Design review of the part built by this model. Coordinates are the model's own, in mm. A direction names the side the tool comes from. Round coordinates to 2 decimals unless told otherwise and drop trailing zeros. Order: outer loops, then holes, each group sorted by start corner. A loop starts at its lowest first (then second) coordinate and runs counter-clockwise, first axis right, second up. Notation, with made-up numbers: (10.5, 4.25) - (15.5, 4.25) arc R25 ccw to (15.5, 38.25) - close; hole circle Ø8 at (-11, 46.5). An arc over 180 degrees is marked (long way). Use CSV: the item, a comma, the result in double quotes.
from build123d import *

# Parameters (mm, degrees)
SKETCH_2_R          = 1.3
EXTRUDE_2_DEPTH     = 3
SKETCH_4_W          = 2
SKETCH_4_H          = 4
EXTRUDE_3_DEPTH     = 6
SKETCH_6_R          = 1.1
CUT_EXTRUDE_2_DEPTH = 45.75


with BuildPart() as part:
    # 草图2 → 凸台-拉伸2 (new body)
    with BuildSketch(Plane.XY):
        with BuildLine():
            ThreePointArc((-3.5, -10), (-2.767766953, -11.767766953), (-1, -12.5))
            Line((-1, -12.5), (50, -12.5))
            ThreePointArc((50, -12.5), (51.767766953, -11.767766953), (52.5, -10))
            Line((52.5, -10), (52.5, 1))
            ThreePointArc((52.5, 1), (51.767766953, 2.767766953), (50, 3.5))
            Line((50, 3.5), (-1, 3.5))
            ThreePointArc((-1, 3.5), (-2.767766953, 2.767766953), (-3.5, 1))
            Line((-3.5, 1), (-3.5, -10))
        make_face()
        with Locations((0, -9)):
            Circle(SKETCH_2_R, mode=Mode.SUBTRACT)
        Circle(SKETCH_2_R, mode=Mode.SUBTRACT)
        with Locations((49, -9)):
            Circle(SKETCH_2_R, mode=Mode.SUBTRACT)
        with Locations((49, 0)):
            Circle(SKETCH_2_R, mode=Mode.SUBTRACT)
    extrude(amount=EXTRUDE_2_DEPTH)

    # 草图4 → 凸台-拉伸3 (add)
    with BuildSketch(Plane.XY.offset(3)):
        with Locations((8.75, 1.5)):
            Rectangle(SKETCH_4_W, SKETCH_4_H)
        with Locations((13.25, 1.5)):
            Rectangle(SKETCH_4_W, SKETCH_4_H)
        with Locations((35.75, 1.5)):
            Rectangle(SKETCH_4_W, SKETCH_4_H)
        with Locations((40.25, 1.5)):
            Rectangle(SKETCH_4_W, SKETCH_4_H)
        with Locations((11.25, -10.5)):
            Rectangle(SKETCH_4_W, SKETCH_4_H)
        with Locations((15.75, -10.5)):
            Rectangle(SKETCH_4_W, SKETCH_4_H)
        with Locations((33.25, -10.5)):
            Rectangle(SKETCH_4_W, SKETCH_4_H)
        with Locations((37.75, -10.5)):
            Rectangle(SKETCH_4_W, SKETCH_4_H)
    extrude(amount=EXTRUDE_3_DEPTH)

    # 草图6 → 切除-拉伸2 (cut, through all)
    with BuildSketch(Plane.ZY.offset(-7.75)):
        with Locations((6, 1.5)):
            Circle(SKETCH_6_R)
        with Locations((6, -10.5)):
            Circle(SKETCH_6_R)
    extrude(amount=-CUT_EXTRUDE_2_DEPTH, mode=Mode.SUBTRACT)


solid = part.part
1) We need section B-B (z = 2.25). Give the boundary of the cut face in (x, y).
Data:
outline,"(-3.5, -10) arc R2.5 ccw to (-1, -12.5) - (50, -12.5) arc R2.5 ccw to (52.5, -10) - (52.5, 1) arc R2.5 ccw to (50, 3.5) - (-1, 3.5) arc R2.5 ccw to (-3.5, 1) - close; hole circle Ø2.6 at (0, -9); hole circle Ø2.6 at (0, 0); hole circle Ø2.6 at (49, -9); hole circle Ø2.6 at (49, 0)"
2) We need section A-A (x = 48.5). Give the boundary of the cut face in (y, z), then the cut area to 3 significant figures.
Data:
outline,"(-12.5, 0) - (-10.2, 0) - (-10.2, 3) - (-12.5, 3) - close; (-7.8, 0) - (-1.2, 0) - (-1.2, 3) - (-7.8, 3) - close; (1.2, 0) - (3.5, 0) - (3.5, 3) - (1.2, 3) - close"
area,"33.6 mm2"
3) We need section D-D (z = 6). Give the number of separate pieces and of enclosed holes in the cut face, then the cut area to 3 significant figures.
Data:
separate pieces,"16"
enclosed holes,"0"
area,"28.8 mm2"
4) We need section C-C (x = 13). Give the boundary of the cut face in (y, z), then the cut area to 3 significant figures.
Data:
outline,"(-12.5, 0) - (3.5, 0) - (3.5, 9) - (-0.5, 9) - (-0.5, 3) - (-12.5, 3) - close; hole circle Ø2.2 at (1.5, 6)"
area,"68.2 mm2"
5) To check wall thickness, follow L1, parallel to X at y = -10.5, z = 7.5; L2, parallel to Y at x = 0, z = 1.7; L3, parallel to Y at x = 8.85, z = 6. State the ranges of each line that lie inside material, in increasing order. Write a range as from..to.
Data:
L1,"x = 10.25..12.25, 14.75..16.75, 32.25..34.25, 36.75..38.75"
L2,"y = -12.5..-10.3, -7.7..-1.3, 1.3..3.5"
L3,"y = -0.5..0.4, 2.6..3.5"
6) The part is to be moulded in two halves that separate along Y. For faces 4 (the face through (40, 2, 9)), 5 (the face through (-2.787, -11.748, 1.479)), 6 (the face through (15.736, -10.921, 7.016)), 7 (the face through (16, -8.5, 6)), say which applies: +Y half, -Y half, draft (parallel to the pull), parting line (faces both ways), or undercut.
Data:
face 4,"draft"
face 5,"-Y half"
face 6,"undercut"
face 7,"+Y half"
7) For faces 1 (the face through (40, -0.5, 6)), 2 (the face through (41.25, 0, 6)), 3 (the face through (39.25, 0, 6)), list the 3-axis set-ups (+Z, -Z, +X, -X, +Y, -Y) from which the entire face can be reached by the end or side of a thin tool; tool diameter is ignored.
Data:
face 1,"+Z, +X, -X, -Y"
face 2,"+Z, +X, +Y, -Y"
face 3,"+Z, +Y, -Y"
8) Insertion check: pin 1 Ø1.2 at (y, z) = (1, 7) entering from -X; pin 2 Ø3 at (y, z) = (2, 5) entering from +X; pin 3 Ø4 at (x, y) = (16.5, 0) entering from -Z; pin 4 Ø1.5 at (x, y) = (23, -5) entering from +Z. Each pin has a flat end and moves straight along its axis. Give the tip position at first contact, or say it passes through.
Data:
pin 1,"stops at x = 7.75"
pin 2,"stops at x = 41.25"
pin 3,"stops at z = 0"
pin 4,"stops at z = 3"
